```python
from build123d import *

# Parameters (mm, degrees)
BOSS_EXTRUDE1_DEPTH          = 3.175
F_10_0_1935_DIAMETER_HOLE2_D = 4.9149
SKETCH8_W                    = 38.1
SKETCH8_H                    = 88.9
CUT_EXTRUDE1_DEPTH           = 3.175
F_10_0_1935_DIAMETER_HOLE3_D = 4.9149


with BuildPart() as part:
    # Sketch1 → Boss-Extrude1 (new body)
    with BuildSketch(Plane(origin=(0, 0, 0), x_dir=(1, 0, 0), z_dir=(0, 1, 0))):
        Polygon((476.25, 581.025), (758.825, 581.025), (758.825, 454.025), (476.25, 454.025), (476.25, 127), (758.825, 127), (758.825, 0), (447.675, 0), (0, 0), (0, 581.025), align=None)
    extrude(amount=BOSS_EXTRUDE1_DEPTH)

    # #10 (0.1935) Diameter Hole2 (through all)
    with Locations(Plane(origin=(0, 3.175, 0), x_dir=(1, 0, 0), z_dir=(0, 1, 0))):
        with Locations((15.875, 455.6125), (15.875, 125.4125), (15.875, 290.5125), (381, 565.15), (381, 15.875), (95.25, 565.15), (95.25, 15.875), (457.2, 125.4125), (457.2, 290.5125), (457.2, 455.6125)):
            Hole(F_10_0_1935_DIAMETER_HOLE2_D / 2)

    # Sketch8 → Cut-Extrude1 (cut)
    with BuildSketch(Plane(origin=(0, 3.175, 0), x_dir=(1, 0, 0), z_dir=(0, 1, 0))):
        with Locations((511.175, 44.45)):
            Rectangle(SKETCH8_W, SKETCH8_H)
        with Locations((511.175, 536.575)):
            Rectangle(SKETCH8_W, SKETCH8_H)
    extrude(amount=-CUT_EXTRUDE1_DEPTH, mode=Mode.SUBTRACT)

    # #10 (0.1935) Diameter Hole3 (through all)
    with Locations(Plane(origin=(0, 3.175, 0), x_dir=(1, 0, 0), z_dir=(0, 1, 0))):
        with Locations((491.8075, 114.3), (542.925, 15.875), (714.375, 15.875), (491.8075, 466.725), (542.925, 565.15), (714.375, 565.15)):
            Hole(F_10_0_1935_DIAMETER_HOLE3_D / 2)


solid = part.part
```
Here's how the part is built. I have some questions about the finished solid (model axes, mm). Round coordinates to 2 decimals unless told otherwise and drop trailing zeros. Write each loop counter-clockwise with the first axis right and the second up, starting at its lowest first coordinate (ties: lowest second). Pieces come first, ordered by that corner, then holes.
Q1. If we section it at B-B on y = 0.8: Give the number of separate pieces and of enclosed holes in the cut face, plus the area to 3 significant figures.
Q2. If we section it at C-C on z = -372: Write out the boundary of the cut face in (x, y) (3 decimals).
Q3. Please list where these lines run through material, in increasing order: probe 1 along X at (y, z) = (2.7, -125) (3 decimals); probe 2 along Z at (x, y) = (457.2, 2.25) (3 decimals); probe 3 along Z at (x, y) = (381, 1.2) (3 decimals).
Q4. Will these pins go through, and if not, where does the flat tip stop? P1, Ø5.5, axis at x = 15.88, z = -455.61, coming from the +Y side (3 decimals); P2, Ø1, axis at x = 520.5, y = 2.5, coming from the +Z side.
Q5. If we section it at A-A on z = -501: Write out the boundary of the cut face in (x, y) (3 decimals).
Answer below:
1. separate pieces: 1
1. enclosed holes: 16
1. area: 341,000 mm2
2. outline: (0, 0) - (476.25, 0) - (476.25, 3.175) - (0, 3.175) - close
3. probe 1: x = 0 to 13.452, 18.298 to 454.777, 459.623 to 758.825
3. probe 2: z = -581.025 to -458.07, -453.155 to -292.97, -288.055 to -127.87, -122.955 to 0
3. probe 3: z = -581.025 to -567.607, -562.693 to -18.332, -13.418 to 0
4. P1: stops at y = 3.175
4. P2: stops at z = -88.9
5. outline: (0, 0) - (492.125, 0) - (492.125, 3.175) - (0, 3.175) - close; (530.225, 0) - (758.825, 0) - (758.825, 3.175) - (530.225, 3.175) - close
